from build123d import *

# Parameters (mm, degrees)
F0_W     = 9.525
F0_H     = 114.3
F1_DEPTH = 76.2
F3_DEPTH = 26.416
F4_DEPTH = 66.294
F5_DEPTH = 25.4
F6_DEPTH = 22.098


with BuildPart() as f1:
    # F0 (on Front) → F1 (new body)
    with BuildSketch(Plane.XZ):
        Polygon((6.5378730087, 113.1293577969), (0, 113.1293577969), (-6.8322808368, 113.1293577969), (-38.1, 36.9293577969), (-28.575, 36.9293577969), (-19.05, 36.9293577969), (-9.525, 36.9293577969), (0, 36.9293577969), (9.525, 36.9293577969), (19.05, 36.9293577969), (28.575, 36.9293577969), (38.1, 36.9293577969), align=None)
        with Locations((-33.3375, -20.2206422031)):
            Rectangle(F0_W, F0_H)
        with Locations((33.3375, -20.2206422031)):
            Rectangle(F0_W, F0_H)
        with Locations((-23.8125, -20.2206422031)):
            Rectangle(F0_W, F0_H)
        with Locations((23.8125, -20.2206422031)):
            Rectangle(F0_W, F0_H)
        with Locations((-14.2875, -20.2206422031)):
            Rectangle(F0_W, F0_H)
        with Locations((14.2875, -20.2206422031)):
            Rectangle(F0_W, F0_H)
        with Locations((-4.7625, -20.2206422031)):
            Rectangle(F0_W, F0_H)
        with Locations((4.7625, -20.2206422031)):
            Rectangle(F0_W, F0_H)
    extrude(amount=F1_DEPTH)

    # F3 (add): a face of the model
    f3_faces = [f1.faces().sort_by_distance(p)[0] for p in [
        (-0.0158753799, -76.2, 4.0859057687),
    ]]
    extrude(f3_faces, amount=-F3_DEPTH)

    # F0 (on Front) → F4 (join)
    with BuildSketch(Plane.XZ):
        Polygon((6.5378730087, 113.1293577969), (0, 113.1293577969), (-6.8322808368, 113.1293577969), (-38.1, 36.9293577969), (-28.575, 36.9293577969), (-19.05, 36.9293577969), (-9.525, 36.9293577969), (0, 36.9293577969), (9.525, 36.9293577969), (19.05, 36.9293577969), (28.575, 36.9293577969), (38.1, 36.9293577969), align=None)
        with Locations((-33.3375, -20.2206422031)):
            Rectangle(F0_W, F0_H)
        with Locations((33.3375, -20.2206422031)):
            Rectangle(F0_W, F0_H)
        with Locations((-23.8125, -20.2206422031)):
            Rectangle(F0_W, F0_H)
        with Locations((23.8125, -20.2206422031)):
            Rectangle(F0_W, F0_H)
        with Locations((-14.2875, -20.2206422031)):
            Rectangle(F0_W, F0_H)
        with Locations((14.2875, -20.2206422031)):
            Rectangle(F0_W, F0_H)
        with Locations((-4.7625, -20.2206422031)):
            Rectangle(F0_W, F0_H)
        with Locations((4.7625, -20.2206422031)):
            Rectangle(F0_W, F0_H)
    extrude(amount=F4_DEPTH)

    # F5 (add): a face of the model
    f5_faces = [f1.faces().sort_by_distance(p)[0] for p in [
        (-38.1, -38.1, -20.2206422031),
    ]]
    extrude(f5_faces, amount=F5_DEPTH)

    # F6 (add): a face of the model
    f6_faces = [f1.faces().sort_by_distance(p)[0] for p in [
        (-9.8283580395, 0, -0.6105930343),
    ]]
    extrude(f6_faces, amount=-F6_DEPTH)


solid = f1.part
Design review of the part built by this model. Coordinates are the model's own, in mm. A direction names the side the tool comes from. Round coordinates to 2 decimals unless told otherwise and drop trailing zeros. Order: outer loops, then holes, each group sorted by start corner. A loop starts at its lowest first (then second) coordinate and runs counter-clockwise, first axis right, second up. Notation, with made-up numbers: M 71,40.5 L 82,40.5 A23 cw 82,59.5 Z; hole C -15,-22.75 d5. An arc over 180 degrees is marked long. Answer as CSV lines item,"result". Start each with the question number.
1) Wall thickness on line 1 along Z through (x, y) = (-50.5, -56.5); line 2 along X through (y, z) = (-59, 63); line 3 along X through (y, z) = (-32, 52): over which ranges is each line inside the solid? List them lowest first. Write a range as [from, to].
2) Tool access review of faces 1 (the face through (-12, -76.2, -5)), 2 (the face through (-51, -38, 36.929)): name each direction out of +Z, -Z, +X, -X, +Y, -Y from which nothing blocks a thin tool from reaching the whole face with its end or side.
3) Add section C-C (z = 71.5). Give the boundary of the cut face in (x, y).
4) Add section B-B (x = -50). Give the boundary of the cut face in (y, z).
5) For pin 1 Ø8 at (x, z) = (4, 25.5) entering from +Y; pin 2 Ø10 at (y, z) = (-27, 71.5) entering from -X; pin 3 Ø8 at (y, z) = (-37, 86.5) entering from +X; pin 4 Ø6 at (x, y) = (20, -13.5) entering from +Z, all flat-tipped, find the tip position at first contact; note any pin that passes through.
6) Add section A-A (y = -29). Give the boundary of the cut face in (x, z).
Resolved:
1,line 1,"[-77.37, 36.93]"
1,line 2,"[-27.4, 27.3]"
1,line 3,"[-31.92, 31.86]"
2,face 1,"+Z, -Z, +X, -X, -Y"
2,face 2,"+Z, -X, +Y, -Y"
3,outline,"M -23.91,-76.2 L 23.78,-76.2 L 23.78,0 L -23.91,0 Z"
4,outline,"M -76.2,-77.37 L 0,-77.37 L 0,36.93 L -76.2,36.93 Z"
5,pin 1,"y = 0"
5,pin 2,"x = -25.97"
5,pin 3,"x = 19.22"
5,pin 4,"z = 87.87"
6,outline,"M -63.5,-77.37 L 38.1,-77.37 L 38.1,36.93 L 6.54,113.13 L -6.83,113.13 L -38.1,36.93 L -63.5,36.93 Z"
